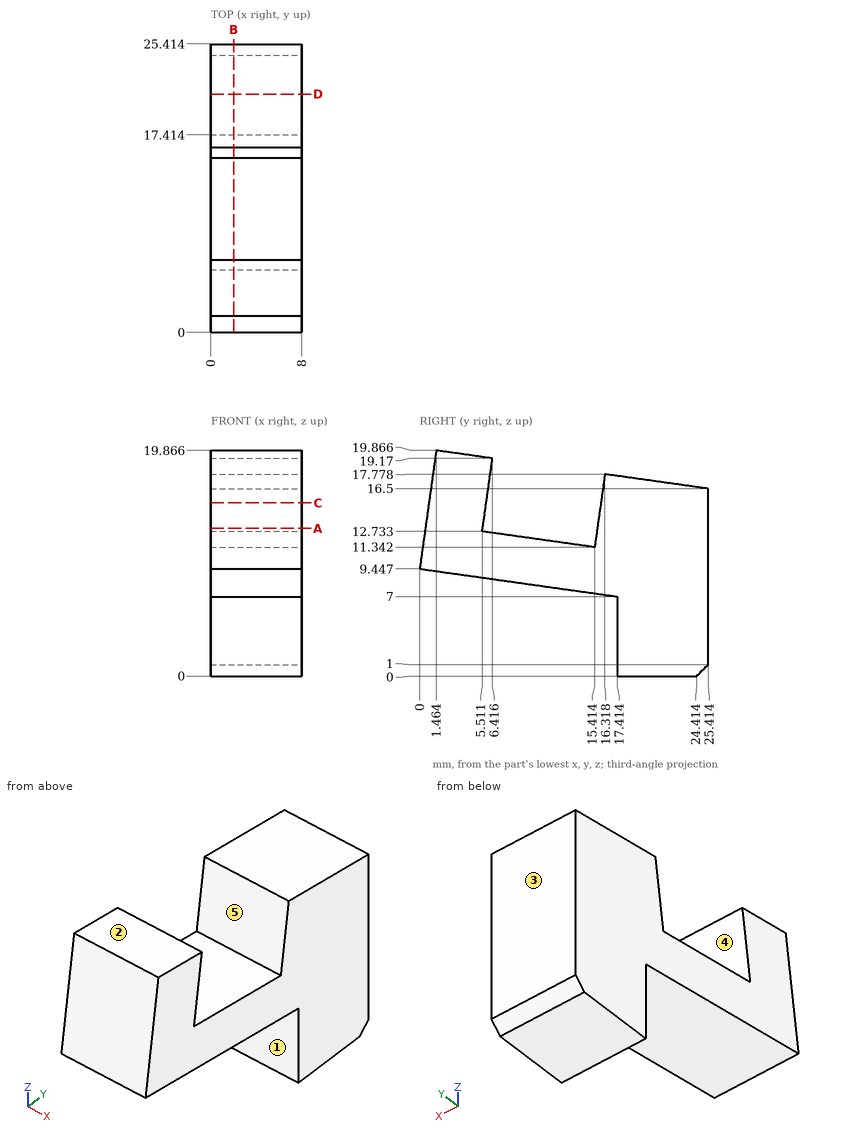
Study the drawing (mm; zero at the part's minimum x, y, z) and answer. A direction names the side the tool comes from. Round coordinates to 2 decimals unless told otherwise and drop trailing zeros. Write each loop counter-clockwise with the first axis right and the second up, starting at its lowest first coordinate (ties: lowest second). Pieces come first, ordered by that corner, then holes.
1) A cutting plane is placed at C-C on z = 15.25. Determine the outline of the cut face in (x, y) (1 decimal).
2) A cutting plane is placed at A-A on z = 13. Determine the outline of the cut face in (x, y).
3) Consider probe 1 along Y at (x, z) = (4.5, 3); probe 2 along Y at (x, z) = (5.25, 13.75) (1 decimal); probe 3 along Z at (x, y) = (3, 8). Determine where each line is inside the solid, lowest interval first.
4) A cutting plane is placed at D-D on y = 21. Determine the outline of the cut face in (x, z), and give its area (3 significant figures).
5) Flat-ended cylindrical pins translate along their axes: P1, Ø4, axis at x = 5.5, y = 10, coming from the +Z side; P2, Ø3, axis at x = 3, z = 2, coming from the -Y side; P3, Ø3, axis at x = 1.5, z = 15, coming from the -Y side; P4, Ø1, axis at y = 16, z = 5, coming from the -X side. Find the tip coordinate at first contact, or state that the pin passes through.
6) Which of the six approach directions +Z, -Z, +X, -X, +Y, -Y give full straight-line access (tool end or side, diameter ignored) to the marked faces 1 and 2?
7) Determine the mould class of the marked faces 3, 4 and 5 for opening direction Z: pulls with the +Z half, pulls with the -Z half, needs draft (parallel to the pull), parting line crosses it, or undercut.
8) A cutting plane is placed at B-B on x = 2. Determine the outline of the cut face in (y, z) (1 decimal), and give its area (3 significant figures).
Entries:
1. outline: (0, 0.8) - (8, 0.8) - (8, 5.9) - (0, 5.9) - close; (0, 16) - (8, 16) - (8, 25.4) - (0, 25.4) - close
2. outline: (0, 0.5) - (8, 0.5) - (8, 5.55) - (0, 5.55) - close; (0, 15.65) - (8, 15.65) - (8, 25.41) - (0, 25.41) - close
3. probe 1: y = 17.41 to 25.41
3. probe 2: y = 0.6 to 5.7, 15.8 to 25.4
3. probe 3: z = 8.32 to 12.38
4. outline: (0, 0) - (8, 0) - (8, 17.12) - (0, 17.12) - close
4. area: 137 mm2
5. P1: stops at z = 12.38
5. P2: stops at y = 17.41
5. P3: stops at y = 0.57
5. P4: passes through
6. face 1: -Z, +X, -X, -Y
6. face 2: +Z, +X, -X, +Y
7. face 3: needs draft
7. face 4: undercut
7. face 5: pulls with the +Z half
8. outline: (0, 9.4) - (17.4, 7) - (17.4, 0) - (24.4, 0) - (25.4, 1) - (25.4, 16.5) - (16.3, 17.8) - (15.4, 11.3) - (5.5, 12.7) - (6.4, 19.2) - (1.5, 19.9) - close
8. area: 248 mm2
